The model under review builds one solid part; all positions refer to its coordinate system, in mm. A direction names the side the tool comes from. Give positions to 0.01 mm unless a question says otherwise; leave off trailing zeros. Order: outer loops, then holes, each group sorted by start corner. A loop starts at its lowest first (then second) coordinate and runs counter-clockwise, first axis right, second up.
```python
from build123d import *

# Parameters (mm, degrees)
F0_W     = 76.2
F0_H     = 38.1
F1_DEPTH = 25.4
F2_SIZE  = 3.175
F3_R     = 9.525
F4_DEPTH = 12.7
F5_SIZE2 = 3.175
F5_SIZE  = 3.175
F6_T     = 7.9375


# Not quite as in the source:
# - a shell that OpenCascade refuses in one call is made with other operations: the cavity is built on its own and cut out


with BuildPart() as f1:
    # F0 (on Top) → F1 (new body)
    with BuildSketch(Plane.XY):
        with Locations((38.1, -19.05)):
            Rectangle(F0_W, F0_H)
    extrude(amount=F1_DEPTH)

    # F2
    f2_edges = [f1.edges().sort_by_distance(p)[0] for p in [
        (38.1, -38.1, 25.4),
        (76.2, -19.05, 25.4),
        (38.1, 0, 25.4),
        (0, -19.05, 25.4),
    ]]
    chamfer(f2_edges, length=F2_SIZE)

    # F3 (on face) → F4 (join)
    with BuildSketch(Plane.XY.offset(25.4)):
        with Locations((19.05, -19.05)):
            Circle(F3_R)
        with Locations((57.15, -19.05)):
            Circle(F3_R)
    extrude(amount=F4_DEPTH)

    # F5
    f5_edges = [f1.edges().sort_by_distance(p)[0] for p in [
        (9.525, -19.05, 38.1),
        (47.625, -19.05, 38.1),
    ]]
    chamfer(f5_edges, length=F5_SIZE, length2=F5_SIZE2)

    # F6: shell of thickness 7.9375, made by hand


with BuildPart() as f6_core1:
    # F6_t2: copy of F1
    add(f1.part)

    # the walls: a layer under each face that stays
    f6_faces = [f6_core1.faces().sort_by_distance(p)[0] for p in [
        (9.525, -19.05, 30.1625),
        (11.1125, -19.05, 36.5125),
        (38.1, -19.05, 25.4),
        (19.05, -19.05, 38.1),
        (38.1, -36.5125, 23.8125),
        (1.5875, -19.05, 23.8125),
        (74.6125, -19.05, 23.8125),
        (38.1, -1.5875, 23.8125),
        (47.625, -19.05, 30.1625),
        (38.1, -38.1, 11.1125),
        (0, -19.05, 11.1125),
        (76.2, -19.05, 11.1125),
        (38.1, 0, 11.1125),
        (49.2125, -19.05, 36.5125),
        (57.15, -19.05, 38.1),
    ]]
    thicken(f6_faces, amount=-F6_T, mode=Mode.SUBTRACT)

    # F6_s3 → F6_t4 (revolve, cut)
    with BuildSketch(Plane.XZ.offset(19.05)):
        Polygon((28.654375, 25.479375), (20.6375, 25.4), (20.6375, 17.4625), (28.575, 17.4625), align=None)
    revolve(axis=Axis((19.05, -19.05, 25.4), (0, 0, 1)), mode=Mode.SUBTRACT)

    # F6_s5 → F6_t6 (revolve, cut)
    with BuildSketch(Plane.XZ.offset(19.05)):
        Polygon((66.754375, 25.479375), (66.675, 17.4625), (58.7375, 17.4625), (58.7375, 25.4), align=None)
    revolve(axis=Axis((57.15, -19.05, 25.4), (0, 0, 1)), mode=Mode.SUBTRACT)


with BuildPart() as f1_1:
    add(f1.part)

    # what is left inside the walls is the cavity
    f6_cavity = [f6_core1.part.solids().sort_by_distance(p)[0] for p in [
        (38.1, -22.754167, 0.079375),
    ]]
    add(f6_cavity, mode=Mode.SUBTRACT)


solid = f1_1.part
```
Item 1: Draft analysis for pull direction Y (two halves, no side actions). For faces 4 (the flat face through (38, 0, 11)), 5 (the flat face through (38, -7.938, 9)), 6 (the flat face through (37.567, -36.49, 23.835)), 7 (the flat face through (0, -19, 11)), state which applies: released by +Y, released by -Y, zero draft, split by the parting line, or undercut.
Values found:
face 4: released by +Y
face 5: undercut
face 6: released by -Y
face 7: zero draft
Item 2: Take a section at B-B (x = 42.5). Give the boundary of the cut face in (y, z) (1 decimal), and give its area (3 significant figures).
Values found:
outline: (-38.1, 0) - (-30.2, 0) - (-30.2, 17.5) - (-7.9, 17.5) - (-7.9, 0) - (0, 0) - (0, 22.2) - (-3.2, 25.4) - (-34.9, 25.4) - (-38.1, 22.2) - close
area: 570 mm2
Item 3: Take a section at A-A (z = 7). Give the boundary of the cut face in (x, y), and give its area (3 significant figures).
Values found:
outline: (0, -38.1) - (76.2, -38.1) - (76.2, 0) - (0, 0) - close; hole (7.94, -30.16) - (68.26, -30.16) - (68.26, -7.94) - (7.94, -7.94) - close
area: 1,560 mm2
Item 4: For faces 1 (the flat face through (57, -19, 30.162)), 2 (the cylindrical face through (17.81, -9.606, 30.096)), 3 (the flat face through (1.61, -19.317, 23.835)), list the 3-axis set-ups (+Z, -Z, +X, -X, +Y, -Y) from which the entire face can be reached by the end or side of a thin tool; tool diameter is ignored.
Values found:
face 1: -Z
face 2: +Z
face 3: +Z, -X, +Y, -Y
Item 5: For line 1 (X direction, y = -19, z = 20); line 2 (X direction, y = -10, z = 10.5); line 3 (X direction, y = -19, z = 23) (3 decimals), list the stretches that pass through material, from the lowest coordinate up.
Values found:
line 1: x = 0 to 17.46, 20.64 to 55.56, 58.74 to 76.2
line 2: x = 0 to 7.94, 68.26 to 76.2
line 3: x = 0.775 to 17.463, 20.637 to 55.563, 58.737 to 75.425
Item 6: Clearance check with flat-ended pins moving along their axes: pin 1 Ø3.5 at (x, y) = (57, -18.5) entering from -Z; pin 2 Ø1 at (x, y) = (19.5, -19.5) entering from -Z. State where each tip first meets the part, or that it passes through.
Values found:
pin 1: stops at z = 17.46
pin 2: stops at z = 30.16
Item 7: Take a section at D-D (z = 36). Give the boundary of the cut face in (x, y).
Values found:
outline: circle Ø16.9 at (19.05, -19.05); circle Ø16.9 at (57.15, -19.05)
